Input: dimensioned drawing with shaded views. Units: mm. Origin: part minimum x, y, z. Coordinates: 2 decimals unless noted, no trailing zeros. Order: outer loops, then holes, each group sorted by start corner. A loop starts at its lowest first (then second) coordinate and runs counter-clockwise, first axis right, second up. Notation, with made-up numbers: (80.25, 64) -> (138.25, 64) arc R22 cw to (138.25, 89) -> close; hole circle Ø10 at (53.5, 9.5). An arc over 180 degrees is marked (long way). Answer in a Markdown table with one row per item. Add a question column.
1) Ray query, line 1 (X direction, y = 154.5, z = 26.5) (1 decimal); line 2 (X direction, y = 586, z = 33.5) (1 decimal); line 3 (Y direction, x = 1699, z = 19) (1 decimal). Return the intervals inside material, ascending. Write a range as from..to.
2) Contact query for flat-ended pins moving along their axis: P1, Ø10, axis at y = 254, z = 16.5, coming from the +X side; P2, Ø8, axis at x = 1473.5, z = 29.5, coming from the -Y side; P3, Ø5, axis at x = 1127.5, z = 26.5, coming from the +Y side. Output: stop coordinate, or through.
3) Section query C-C on x = 479. Return the cut outline in (y, z).
4) Section query A-A on z = 22. Return the cut outline in (x, y), then the cut area to 3 significant figures.
5) Section query B-B on y = 287. Return the cut outline in (x, z), then the cut area to 3 significant figures.
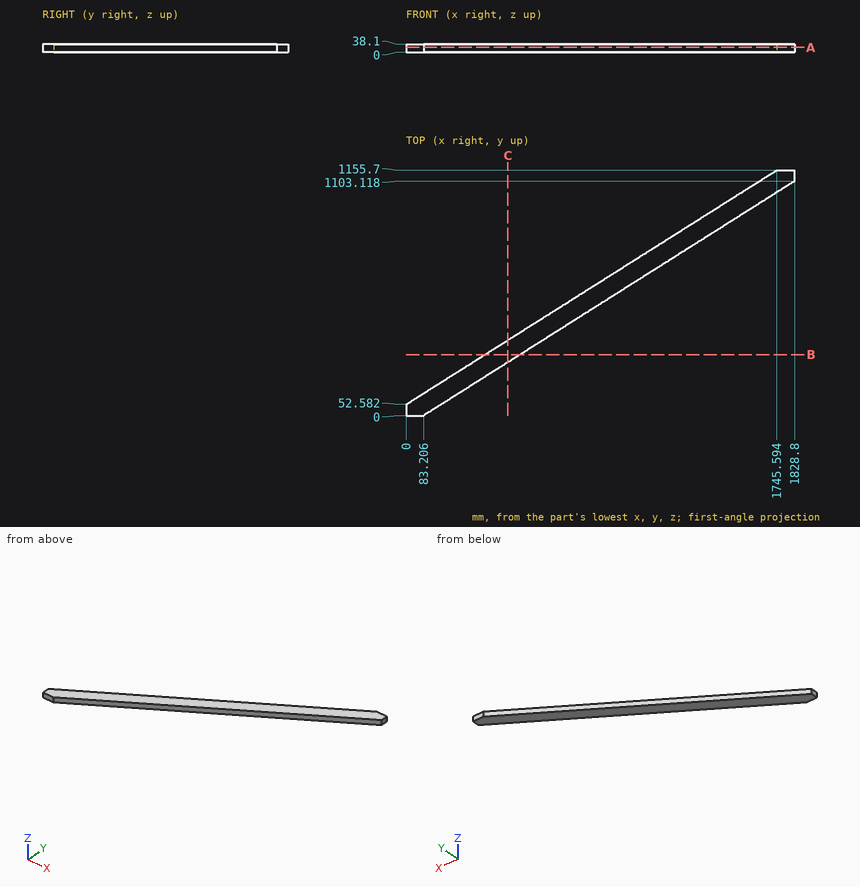
Result:
| question | item | result |
|---|---|---|
| 1 | line 1 | 161.3..327.7 |
| 1 | line 2 | 844.1..1010.5 |
| 1 | line 3 | 1021.1..1126.3 |
| 2 | P1 | x = 493.05 |
| 2 | P2 | y = 876.06 |
| 2 | P3 | y = 766.68 |
| 3 | outline | (250.12, 0) -> (355.28, 0) -> (355.28, 38.1) -> (250.12, 38.1) -> close |
| 4 | outline | (0, 0) -> (83.21, 0) -> (1828.8, 1103.12) -> (1828.8, 1155.7) -> (1745.59, 1155.7) -> (0, 52.58) -> close |
| 4 | area | 188,000 mm2 |
| 5 | outline | (370.95, 0) -> (537.36, 0) -> (537.36, 38.1) -> (370.95, 38.1) -> close |
| 5 | area | 6,340 mm2 |
